from build123d import *

# Parameters (mm, degrees)
F0_R     = 285.75
F1_DEPTH = 917.575
F2_R     = 266.7
F3_DEPTH = 889
F4_R     = 30.48
F5_DEPTH = 547.83055
F6_R     = 30.48
F7_DEPTH = 651.82147


with BuildPart() as f1:
    # F0 (on Top) → F1 (new body)
    with BuildSketch(Plane.XY):
        Circle(F0_R)
    extrude(amount=F1_DEPTH)

    # F2 (on face) → F3 (cut)
    with BuildSketch(Plane.XY.offset(917.575)):
        Circle(F2_R)
    extrude(amount=-F3_DEPTH, mode=Mode.SUBTRACT)

    # F4 (on Right) → F5 (cut)
    with BuildSketch(Plane.YZ):
        with Locations((0, 739.775)):
            Circle(F4_R)
    extrude(amount=F5_DEPTH, mode=Mode.SUBTRACT)

    # F6 (on Right) → F7 (cut)
    with BuildSketch(Plane.YZ):
        with Locations((81.008007, 76.2)):
            Circle(F6_R)
        with Locations((-96.791993, 76.2)):
            Circle(F6_R)
    extrude(amount=-F7_DEPTH, mode=Mode.SUBTRACT)


solid = f1.part
Can you work these out from the model? Positions are in its coordinate system, mm. A direction names the side the tool comes from. Give positions to 0.01 mm unless a question says otherwise; leave off trailing zeros. Write each loop counter-clockwise with the first axis right and the second up, starting at its lowest first coordinate (ties: lowest second). Pieces come first, ordered by that corner, then holes. Notation, with made-up numbers: (21.25, 28.25) -> (59.25, 28.25) arc R6 ccw to (59.25, 34.25) -> close; hole circle Ø1 at (69, 1.25). An arc over 180 degrees is marked (long way). Answer as a JSON object with one key per item and string values. Group by question number.
Item 1: Suppose I cut it at C-C (x = 0). Please give me the cut outline in (y, z) (3 decimals), plus the area to 3 significant figures.
Item 2: We'd pull the mould along X, two halves only. Please class faces 1 (the face through (-234.2, 128.3, 917.575)), 2 (the face through (-285.474, 12.564, 452.364)), 3 (the face through (-4, 4, 28.575)), 4 (the face through (254.384, 80.109, 479.298)): +X half, -X half, draft (parallel to the pull), parting line (faces both ways), or undercut.
Item 3: Suppose I cut it at D-D (z = 76.2). Please give me the cut outline in (x, y), plus the area to 3 significant figures.
Item 4: Please list where these lines run through material, in increasing order: line 1 (Z direction, x = 277.75, y = 0) (3 decimals); line 2 (Y direction, x = 0, z = 489); line 3 (Z direction, x = 8, y = -109) (3 decimals). Write a range as [from, to].
Item 5: I'm going to push flat-ended pins straight in: P1, Ø12, axis at x = -52, z = 500, coming from the -Y side; P2, Ø1.5, axis at y = 117, z = 762, coming from the -X side; P3, Ø3, axis at x = 206.5, z = 664.5, coming from the +Y side. Where does each tip first touch, or does it pass through?
Item 6: Suppose I cut it at B-B (z = 305). Please give me the cut outline in (x, y).
Item 7: Suppose I cut it at A-A (y = 0). Please give me the cut outline in (x, z) (3 decimals).
Item 8: For faces 5 (the face through (-261.491, 97.394, 101.901)), 6 (the face through (-4, 4, 0)), 7 (the face through (275.21, -30.45, 741.12)), which set-ups out of +Z, -Z, +X, -X, +Y, -Y let a thin tool reach every point of the face, with its end or its side?
Findings:
{
 "1": {"outline": "(-285.75, 0) -> (285.75, 0) -> (285.75, 917.575) -> (266.7, 917.575) -> (266.7, 28.575) -> (-266.7, 28.575) -> (-266.7, 917.575) -> (-285.75, 917.575) -> close", "area": "50,200 mm²"},
 "2": {"face 1": "draft", "face 2": "parting line", "face 3": "undercut", "face 4": "undercut"},
 "3": {"outline": "(-281.25, 50.53) arc R285.75 ccw to (-277.95, -66.31) -> (-258.32, -66.31) arc R266.7 cw to (-261.87, 50.53) -> close; (-263.1, 111.49) -> (-242.28, 111.49) arc R266.7 cw (long way) to (-234.37, -127.27) -> (-255.84, -127.27) arc R285.75 ccw (long way) to start", "area": "30,600 mm²"},
 "4": {"line 1": "z = [0, 709.295], [770.255, 917.575]", "line 2": "y = [-285.75, -266.7], [266.7, 285.75]", "line 3": "z = [0, 28.575]"},
 "5": {"P1": "stops at y = -282.02", "P2": "stops at x = -261.03", "P3": "stops at y = 199.07"},
 "6": {"outline": "circle Ø571.5 at (0, 0); hole circle Ø533.4 at (0, 0)"},
 "7": {"outline": "(-285.75, 0) -> (285.75, 0) -> (285.75, 709.295) -> (266.7, 709.295) -> (266.7, 28.575) -> (-266.7, 28.575) -> (-266.7, 917.575) -> (-285.75, 917.575) -> close; (266.7, 770.255) -> (285.75, 770.255) -> (285.75, 917.575) -> (266.7, 917.575) -> close"},
 "8": {"face 5": "-X", "face 6": "-Z, +X, -X, +Y, -Y", "face 7": "+X"}
}
